Geometry: final body of the model. Coordinates: model frame, mm. Face numbers are marked on the shaded views. A direction names the side the tool comes from. Round coordinates to 2 decimals unless told otherwise and drop trailing zeros. Loops run counter-clockwise (first coordinate to the right, second up) from the corner with the lowest first, then second, coordinate; pieces in that order, holes last. Notation, with made-up numbers: M 28.25,71.25 L 39.25,71.25 A18 cw 39.25,90.25 Z; hole C -37,81 d1. An arc over 180 degrees is marked long. Answer as a JSON object with one key per item and string values.
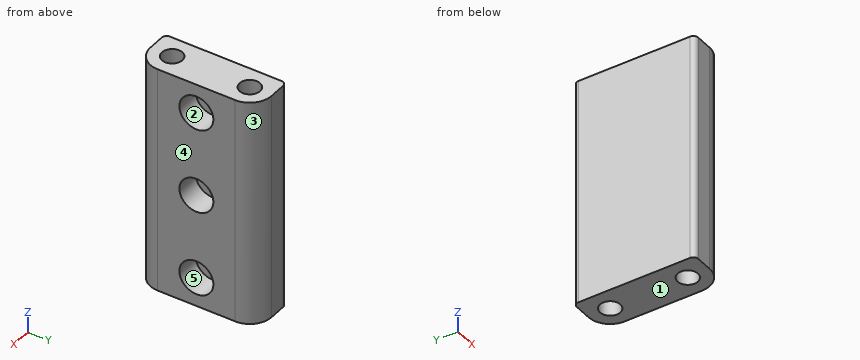
```python
from build123d import *

# Parameters (mm, degrees)
BOSS_EXTRUDE1_DEPTH = 47
SKETCH2_R           = 2.1
CUT_EXTRUDE1_DEPTH  = 4
SKETCH3_R           = 2.1
CUT_EXTRUDE2_DEPTH  = 4
SKETCH4_R           = 3.5
CUT_EXTRUDE3_DEPTH  = 5
FILLET1_R           = 1


with BuildPart() as part:
    # Sketch1 → Boss-Extrude1 (new body)
    with BuildSketch(Plane.XY):
        with BuildLine():
            Line((-4.5, -4.5), (-4.5, 20.5))
            Line((-4.5, 20.5), (0, 20.5))
            ThreePointArc((0, 20.5), (3.181980515, 19.181980515), (4.5, 16))
            Line((4.5, 16), (4.5, 0))
            ThreePointArc((4.5, 0), (3.181980515, -3.181980515), (0, -4.5))
            Line((0, -4.5), (-4.5, -4.5))
        make_face()
    extrude(amount=BOSS_EXTRUDE1_DEPTH)

    # Sketch2 → Cut-Extrude1 (cut)
    with BuildSketch(Plane.XY.offset(47)):
        with Locations((0, 16)):
            Circle(SKETCH2_R)
        Circle(SKETCH2_R)
    extrude(amount=-CUT_EXTRUDE1_DEPTH, mode=Mode.SUBTRACT)

    # Sketch3 → Cut-Extrude2 (cut)
    with BuildSketch(Plane(origin=(0, 0, 0), x_dir=(-1, 0, 0), z_dir=(0, 0, -1))):
        Circle(SKETCH3_R)
        with Locations((0, 16)):
            Circle(SKETCH3_R)
    extrude(amount=-CUT_EXTRUDE2_DEPTH, mode=Mode.SUBTRACT)

    # Sketch4 → Cut-Extrude3 (cut)
    with BuildSketch(Plane(origin=(4.5, 0, 0), x_dir=(0, 0, -1), z_dir=(1, 0, 0))):
        with Locations((-41, 8)):
            Circle(SKETCH4_R)
        with Locations((-23.5, 8)):
            Circle(SKETCH4_R)
        with Locations((-6, 8)):
            Circle(SKETCH4_R)
    extrude(amount=-CUT_EXTRUDE3_DEPTH, mode=Mode.SUBTRACT)

    # Fillet1
    fillet1_edges = [part.edges().sort_by_distance(p)[0] for p in [
        (-4.5, -4.5, 23.5),
        (-4.5, 20.5, 23.5),
    ]]
    fillet(fillet1_edges, radius=FILLET1_R)


solid = part.part
```
1) Cut plane A-A on z = 18. Return the cut outline in (x, y).
Geometry results:
{"outline": "M -4.5,-3.5 A1 ccw -3.5,-4.5 L 0,-4.5 A4.5 ccw 4.5,0 L 4.5,16 A4.5 ccw 0,20.5 L -3.5,20.5 A1 ccw -4.5,19.5 Z"}
2) Set-up query: the marked faces 1 and 2. Return all of +Z, -Z, +X, -X, +Y, -Y with unobstructed straight access to the full face (end or side cutting, diameter ignored); none if empty.
Geometry results:
{"face 1": "-Z, +X, -X, +Y, -Y", "face 2": "+X"}
3) Cut plane C-C on x = 3. Return the cut outline in (y, z), and give its area (3 significant figures).
Geometry results:
{"outline": "M -3.35,0 L 19.35,0 L 19.35,47 L -3.35,47 Z; hole C 8,6 d7; hole C 8,23.5 d7; hole C 8,41 d7", "area": "952 mm2"}
4) Cut plane D-D on z = 6. Return the cut outline in (x, y), and give its area (3 significant figures).
Geometry results:
{"outline": "M -4.5,-3.5 A1 ccw -3.5,-4.5 L 0,-4.5 A4.5 ccw 4.5,0 L 4.5,4.5 L -0.5,4.5 L -0.5,11.5 L 4.5,11.5 L 4.5,16 A4.5 ccw 0,20.5 L -3.5,20.5 A1 ccw -4.5,19.5 Z", "area": "181 mm2"}
5) First-contact query: pin 1 (2.5 mm diameter, centred on x = 0, y = 16, fed in from +Z); pin 2 (3 mm diameter, centred on x = 2, z = 6.5, fed in from -Y); pin 3 (6.5 mm diameter, centred on y = 8, z = 6, fed in from +X). Flat tips, straight axial feed; report the tip coordinate or a pass-through.
Geometry results:
{"pin 1": "z = 43", "pin 2": "y = -4.47", "pin 3": "x = -0.5"}
6) Line query: probe 1 along Z at (x, y) = (3.5, 7.5); probe 2 along Y at (x, z) = (0.75, 39); probe 3 along X at (y, z) = (6.5, 8). Output: solid intervals per line, ascending.
Geometry results:
{"probe 1": "0 to 2.54, 9.46 to 20.04, 26.96 to 37.54, 44.46 to 47", "probe 2": "-4.44 to 5.13, 10.87 to 20.44", "probe 3": "-4.5 to -0.5"}
7) Cut plane B-B on y = 8. Return the cut outline in (x, z).
Geometry results:
{"outline": "M -4.5,0 L 4.5,0 L 4.5,2.5 L -0.5,2.5 L -0.5,9.5 L 4.5,9.5 L 4.5,20 L -0.5,20 L -0.5,27 L 4.5,27 L 4.5,37.5 L -0.5,37.5 L -0.5,44.5 L 4.5,44.5 L 4.5,47 L -4.5,47 Z"}
8) Pull-direction query (Y, two-part tool) for the marked faces 3, 4 and 5; classes: +Y half, -Y half, draft (parallel to the pull), parting line (faces both ways), or undercut.
Geometry results:
{"face 3": "+Y half", "face 4": "draft", "face 5": "undercut"}
